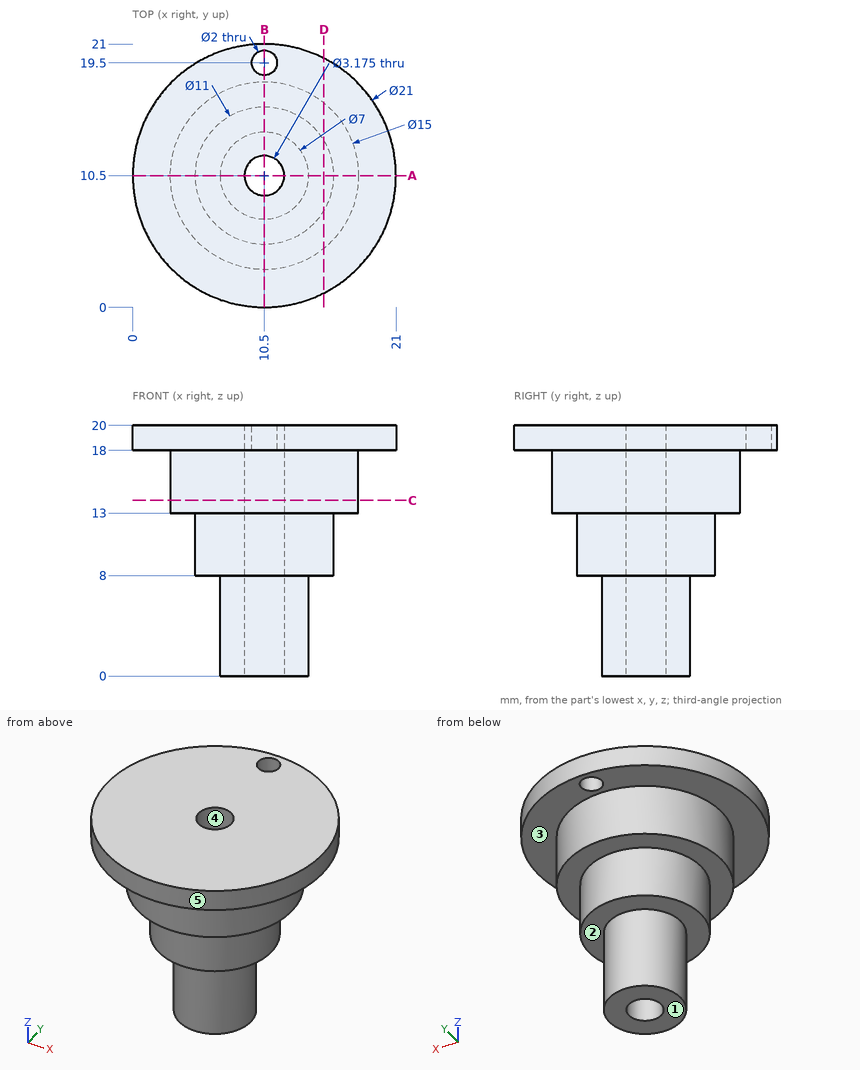
Can you work these out from the drawing? Everything is in mm from the part's minimum corner. A direction names the side the tool comes from. Round coordinates to 2 decimals unless told otherwise and drop trailing zeros. Loops run counter-clockwise (first coordinate to the right, second up) from the corner with the lowest first, then second, coordinate; pieces in that order, holes last. Notation, with made-up numbers: (-21.5, 57) -> (-12.5, 57) arc R20 ccw to (-12.5, 61) -> close; hole circle Ø9 at (59, 72.5). An arc over 180 degrees is marked (long way). One line per question, with ' | ' between items.
(1) If we section it at C-C on z = 14: List the corners of the cut face in (x, y) for me (1 decimal), and give its area (3 significant figures).
Model answer:
outline: circle Ø15 at (10.5, 10.5); hole circle Ø3.2 at (10.5, 10.5) | area: 169 mm^2
(2) For the marked faces 1 and 2, which set-ups out of +Z, -Z, +X, -X, +Y, -Y let a thin tool reach every point of the face, with its end or its side?
Model answer:
face 1: -Z, +X, -X, +Y, -Y | face 2: -Z
(3) If we section it at B-B on x = 10.5: List the corners of the cut face in (y, z) for me.
Model answer:
outline: (0, 18) -> (3, 18) -> (3, 13) -> (5, 13) -> (5, 8) -> (7, 8) -> (7, 0) -> (8.91, 0) -> (8.91, 20) -> (0, 20) -> close; (12.09, 0) -> (14, 0) -> (14, 8) -> (16, 8) -> (16, 13) -> (18, 13) -> (18, 18) -> (18.5, 18) -> (18.5, 20) -> (12.09, 20) -> close; (20.5, 18) -> (21, 18) -> (21, 20) -> (20.5, 20) -> close
(4) If I drill on probe 1 along Y at (x, z) = (10.5, 18.9); probe 2 along Y at (x, z) = (10.5, 12.5); probe 3 along Z at (x, y) = (7.5, 15.75), over which ranges is the centre line in solid material (lowest first)?
Model answer:
probe 1: y = 0 to 8.91, 12.09 to 18.5, 20.5 to 21 | probe 2: y = 5 to 8.91, 12.09 to 16 | probe 3: z = 13 to 20
(5) If we section it at A-A on y = 10.5: List the corners of the cut face in (x, z) for me.
Model answer:
outline: (0, 18) -> (3, 18) -> (3, 13) -> (5, 13) -> (5, 8) -> (7, 8) -> (7, 0) -> (8.91, 0) -> (8.91, 20) -> (0, 20) -> close; (12.09, 0) -> (14, 0) -> (14, 8) -> (16, 8) -> (16, 13) -> (18, 13) -> (18, 18) -> (21, 18) -> (21, 20) -> (12.09, 20) -> close
(6) Thinking about a two-plate mould opening in X: for the marked faces 3, 4 and 5, which applies, released by +X, released by -X, zero draft, split by the parting line, or undercut?
Model answer:
face 3: zero draft | face 4: undercut | face 5: split by the parting line
(7) If we section it at D-D on x = 15.25: List the corners of the cut face in (y, z) for me, and give its area (3 significant figures).
Model answer:
outline: (1.14, 18) -> (4.7, 18) -> (4.7, 13) -> (7.73, 13) -> (7.73, 8) -> (13.27, 8) -> (13.27, 13) -> (16.3, 13) -> (16.3, 18) -> (19.86, 18) -> (19.86, 20) -> (1.14, 20) -> close | area: 123 mm^2
(8) For pin 1 Ø4 at (x, y) = (3, 8) entering from -Z; pin 2 Ø3 at (x, z) = (11, 13) entering from -Y; pin 3 Ø10 at (x, z) = (14.5, 7.5) entering from +Y, each with a flat end and sliding along its axis, tell me the tip position at first contact or that it passes through.
Model answer:
pin 1: stops at z = 13 | pin 2: stops at y = 3 | pin 3: stops at y = 16
